from build123d import *

# Parameters (mm, degrees)
SKETCH_1_W          = 30
SKETCH_1_H          = 30
EXTRUDE_1_DEPTH     = 9
SKETCH_2_W          = 5.7
SKETCH_2_H          = 30
EXTRUDE_2_DEPTH     = 30
CUT_EXTRUDE_START   = -30
CUT_EXTRUDE_2_DEPTH = 30
SKETCH_4_R          = 4
CUT_EXTRUDE_3_DEPTH = 52.439284598
SKETCH_5_R          = 8
CUT_EXTRUDE_4_DEPTH = 2
SKETCH_6_R          = 4
CUT_EXTRUDE_5_DEPTH = 37.742346142
SKETCH_7_W          = 8.2
SKETCH_7_H          = 1
EXTRUDE_3_DEPTH     = 2


# Read off the part's stored shape, not the designer's step: 切除-拉伸2
with BuildPart() as part:
    # 草图1 → 凸台-拉伸1 (new body)
    with BuildSketch(Plane.XY):
        Rectangle(SKETCH_1_W, SKETCH_1_H)
    extrude(amount=EXTRUDE_1_DEPTH)

    # 草图2 → 凸台-拉伸2 (add)
    with BuildSketch(Plane.XY.offset(9)):
        with Locations((-12.15, 0)):
            Rectangle(SKETCH_2_W, SKETCH_2_H)
        with Locations((12.15, 0)):
            Rectangle(SKETCH_2_W, SKETCH_2_H)
    extrude(amount=EXTRUDE_2_DEPTH)

    # 切除-拉伸2 outline → 切除-拉伸2 (cut)
    with BuildSketch(Plane.ZY.offset(15).offset(CUT_EXTRUDE_START)):
        with BuildLine():
            Line((39, 15), (24, 15))
            ThreePointArc((24, 15), (34.606601718, 10.606601718), (39, 0))
            Line((39, 0), (39, 15))
        make_face()
        with BuildLine():
            Line((39, -15), (39, 0))
            ThreePointArc((39, 0), (34.606601718, -10.606601718), (24, -15))
            Line((24, -15), (39, -15))
        make_face()
    extrude(amount=CUT_EXTRUDE_2_DEPTH, mode=Mode.SUBTRACT)

    # 草图4 → 切除-拉伸3 (cut, through all)
    with BuildSketch(Plane.ZY.offset(15)):
        with Locations((24, 0)):
            Circle(SKETCH_4_R)
    extrude(amount=-CUT_EXTRUDE_3_DEPTH, mode=Mode.SUBTRACT)

    # 草图5 → 切除-拉伸4 (cut)
    with BuildSketch(Plane.ZY.offset(15)):
        with Locations((24, 0)):
            Circle(SKETCH_5_R)
    extrude(amount=-CUT_EXTRUDE_4_DEPTH, mode=Mode.SUBTRACT)

    # 草图6 → 切除-拉伸5 (cut, through all)
    with BuildSketch(Plane.XY.offset(9)):
        Circle(SKETCH_6_R)
    extrude(amount=-CUT_EXTRUDE_5_DEPTH, mode=Mode.SUBTRACT)

    # 草图7 → 凸台-拉伸3 (add)
    with BuildSketch(Plane(origin=(0, 0, 0), x_dir=(-1, 0, 0), z_dir=(0, 0, -1))):
        with Locations((0, 14.5)):
            Rectangle(SKETCH_7_W, SKETCH_7_H)
        with Locations((0, -14.5)):
            Rectangle(SKETCH_7_W, SKETCH_7_H)
    extrude(amount=EXTRUDE_3_DEPTH)


solid = part.part
Read the model definition and answer for the solid it produces. Units are mm, in the model's axes. A direction names the side the tool comes from. Coordinates: 2 decimals unless noted, no trailing zeros. Order: outer loops, then holes, each group sorted by start corner. A loop starts at its lowest first (then second) coordinate and runs counter-clockwise, first axis right, second up. Notation, with made-up numbers: M 77,75 L 119,75 A21 cw 119,101 Z; hole C -36,19.25 d10. An arc over 180 degrees is marked long. Put each result on its own line as item: value. Start each with the question number.
Item 1: Consider probe 1 along X at (y, z) = (8.25, 11); probe 2 along Y at (x, z) = (12.05, 24); probe 3 along Z at (x, y) = (9, 11.75). Determine where each line is inside the solid, lowest interval first. Write a range as [from, to].
Item 2: Given pin 1 Ø0.5 at (y, z) = (-14.5, -0.5) entering from +X; pin 2 Ø4 at (x, y) = (4, -6.5) entering from +Z; pin 3 Ø6.5 at (x, y) = (0, 0) entering from -Z; pin 4 Ø4 at (x, y) = (-10, 0) entering from -Z, each flat-ended and moving along its own axis, determine where each tip first touches the part or whether it passes through.
Item 3: Section D-D, the plane y = -0.5 is taken. Determine the outline of the cut face in (x, z), plus the area to 3 significant figures.
Item 4: The mould has two halves that part along Y. Classify faces 1 (the face through (0, 15, 8)), 2 (the face through (-14.014, -4.868, 17.651)), 3 (the face through (9.3, 3, 20)): +Y half, -Y half, draft (parallel to the pull), parting line (faces both ways), or undercut.
Item 5: Section C-C, the plane z = 22 is taken. Determine the outline of the cut face in (x, y).
Item 6: For faces 4 (the face through (-13, -2, 20)), 5 (the face through (4.1, 14.5, -1)), 6 (the face through (-4.1, -14.5, -1)), 7 (the face through (0, -14, -1)), 8 (the face through (-2, 4, 9)), determine the directions among +Z, -Z, +X, -X, +Y, -Y from which every point of the face is accessible in a straight line to the end or side of a thin tool.
Item 7: Section B-B, the plane x = 0 is taken. Determine the outline of the cut face in (y, z), plus the area to 3 significant figures.
Item 8: Section A-A, the plane z = 12.5 is taken. Determine the outline of the cut face in (x, y), plus the area to 3 significant figures.
Computed:
1. probe 1: x = [-15, -9.3], [9.3, 15]
1. probe 2: y = [-15, -4], [4, 15]
1. probe 3: z = [0, 9]
2. pin 1: stops at x = 4.1
2. pin 2: stops at z = 9
2. pin 3: passes through
2. pin 4: stops at z = 0
3. outline: M -15,0 L -3.97,0 L -3.97,9 L -9.3,9 L -9.3,20.03 L -13,20.03 L -13,16.02 L -15,16.02 Z; M -15,31.98 L -13,31.98 L -13,27.97 L -9.3,27.97 L -9.3,38.99 L -15,38.99 Z; M 3.97,0 L 15,0 L 15,20.03 L 9.3,20.03 L 9.3,9 L 3.97,9 Z; M 9.3,27.97 L 15,27.97 L 15,38.99 L 9.3,38.99 Z
3. area: 434 mm2
4. face 1: +Y half
4. face 2: undercut
4. face 3: draft
5. outline: M -15,-15 L -9.3,-15 L -9.3,-3.46 L -13,-3.46 L -13,-7.75 L -15,-7.75 Z; M -15,7.75 L -13,7.75 L -13,3.46 L -9.3,3.46 L -9.3,15 L -15,15 Z; M 9.3,-15 L 15,-15 L 15,-3.46 L 9.3,-3.46 Z; M 9.3,3.46 L 15,3.46 L 15,15 L 9.3,15 Z
6. face 4: -X
6. face 5: -Z, +X, +Y, -Y
6. face 6: -Z, -X, +Y, -Y
6. face 7: -Z, +X, -X
6. face 8: +Z, +Y, -Y
7. outline: M -15,-2 L -14,-2 L -14,0 L -4,0 L -4,9 L -15,9 Z; M 4,0 L 14,0 L 14,-2 L 15,-2 L 15,9 L 4,9 Z
7. area: 202 mm2
8. outline: M -15,-15 L -9.3,-15 L -9.3,15 L -15,15 Z; M 9.3,-15 L 15,-15 L 15,15 L 9.3,15 Z
8. area: 342 mm2
